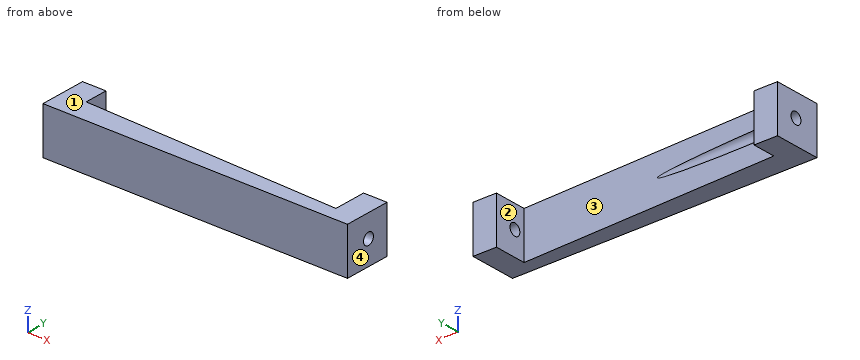
```python
from build123d import *

# Parameters (mm, degrees)
F1_DEPTH = 25.4
F3_D     = 6.35


with BuildPart() as f1:
    # F0 (on Top) → F1 (new body)
    with BuildSketch(Plane.XY):
        Polygon((-94.18092, 50.48936), (-106.88092, 50.48936), (-106.88092, 25.08936), (58.21908, 25.08936), (58.21908, 50.48936), (45.51908, 50.48936), (45.51908, 32.70936), (-94.18092, 37.78936), align=None)
    extrude(amount=F1_DEPTH)

    # F3 (through all)
    with Locations(Plane.YZ.offset(58.21908)):
        with Locations((38.594734, 13.081748)):
            Hole(F3_D / 2)


solid = f1.part
```
For this review, take the finished solid that the model builds, in its own axes (mm). Face numbers are marked on the shaded views. Coordinates: 2 decimals unless noted, no trailing zeros. Write each loop counter-clockwise with the first axis right and the second up, starting at its lowest first coordinate (ties: lowest second). Pieces come first, ordered by that corner, then holes. Notation, with made-up numbers: (47, 13) -> (89, 13) arc R20 ccw to (89, 27) -> close; hole circle Ø10 at (61, 31). An arc over 180 degrees is marked (long way). Put each result on its own line as item: value.
Q1. Wall thickness on L1, parallel to X at y = 42.5, z = 10.5; L2, parallel to Y at x = -58.5, z = 12.75; L3, parallel to Y at x = -21.5, z = 19.5: over which ranges is each line inside the solid? List them lowest first.
From the geometry:
L1: x = -106.88 to -94.18, 45.52 to 58.22
L2: y = 25.09 to 35.44
L3: y = 25.09 to 35.15
Q2. Clearance check with flat-ended pins moving along their axes: pin 1 Ø3 at (x, z) = (-13.5, 16) entering from +Y; pin 2 Ø5 at (x, y) = (-60, 41) entering from +Z. State where each tip first meets the part, or that it passes through.
From the geometry:
pin 1: stops at y = 34.91
pin 2: passes through
Q3. Take a section at D-D, the plane x = 33. State the section outline as (y, z) points.
From the geometry:
outline: (25.09, 0) -> (33.16, 0) -> (33.16, 25.4) -> (25.09, 25.4) -> close
Q4. Take a section at A-A, the plane y = 49. State the section outline as (x, z) points, then the cut area to 3 significant figures.
From the geometry:
outline: (-106.88, 0) -> (-94.18, 0) -> (-94.18, 25.4) -> (-106.88, 25.4) -> close; (45.52, 0) -> (58.22, 0) -> (58.22, 25.4) -> (45.52, 25.4) -> close
area: 645 mm2
Q5. The part is to be moulded in two halves that separate along X. For the marked faces 1, 2, 3 and 4, say which applies: +X half, -X half, draft (parallel to the pull), parting line (faces both ways), or undercut.
From the geometry:
face 1: draft
face 2: undercut
face 3: undercut
face 4: +X half
Q6. Take a section at B-B, the plane x = -56. State the section outline as (y, z) points (3 decimals).
From the geometry:
outline: (25.089, 0) -> (36.401, 0) -> (36.401, 10.787) arc R3.175 cw to (36.401, 15.377) -> (36.401, 25.4) -> (25.089, 25.4) -> close
